Answer from the drawing. Dimensions are ordinates in mm from the lowest x, y and z of the part. A direction names the side the tool comes from. Give positions to 0.01 mm unless a question says otherwise; leave off trailing zeros. Loops run counter-clockwise (first coordinate to the right, second up) from the corner with the lowest first, then second, coordinate; pieces in that order, holes last.
Item 1: A tool of negligible diameter and unlimited length cuts with its end or side. For the marked faces 4 and 5, from which of +Z, -Z, +X, -X, +Y, -Y can it reach the whole face along a straight path? Write none if from no direction.
Item 2: Section B-B, the plane y = 58.5 is taken. Give the vertices of the cut face in (x, z).
Item 3: Consider line 1 along Y through (x, z) = (2.25, 8); line 2 along Z through (x, y) = (4.75, 51.5); line 3 along Z through (x, y) = (9.5, 40.5). Determine where each line is inside the solid, lowest interval first.
Item 4: Each of these flat-tipped pins is pushed along its axis until it touches: pin 1 Ø4 at (y, z) = (68.5, 6.5) entering from +X; pin 2 Ø3 at (y, z) = (51.5, 2) entering from +X; pin 3 Ø1 at (y, z) = (59.5, 1.5) entering from +X. Where does it stop, or does it pass through?
Item 5: Section A-A, the plane z = 5 is taken. Give the vertices of the cut face in (x, y), and give its area (3 significant figures).
Item 6: The mould has two halves that part along Y. Classify the marked faces 1, 2 and 3: pulls with the +Y half, pulls with the -Y half, needs draft (parallel to the pull), parting line crosses it, or undercut.
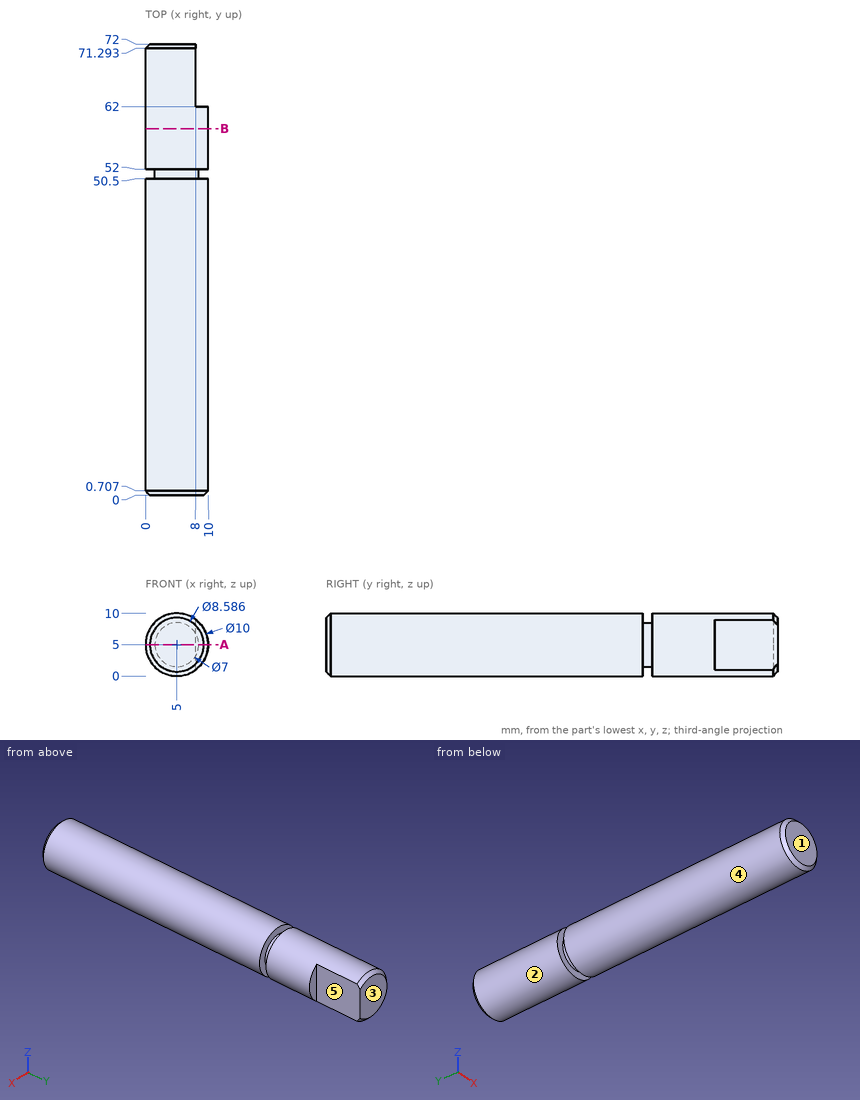
Worked answers:
1. face 4: +Y, -Y
1. face 5: +Z, -Z, +X, +Y
2. outline: circle Ø10 at (5, 5)
3. line 1: y = 0 to 50.5, 52 to 72
3. line 2: z = 1.51 to 8.49
3. line 3: z = 2.82 to 7.18
4. pin 1: stops at x = 8
4. pin 2: stops at x = 9.74
4. pin 3: stops at x = 9
5. outline: (0, 0.71) - (0.71, 0) - (9.29, 0) - (10, 0.71) - (10, 50.5) - (8.5, 50.5) - (8.5, 52) - (10, 52) - (10, 62) - (8, 62) - (8, 72) - (0.71, 72) - (0, 71.29) - (0, 52) - (1.5, 52) - (1.5, 50.5) - (0, 50.5) - close
5. area: 695 mm2
6. face 1: pulls with the -Y half
6. face 2: needs draft
6. face 3: pulls with the +Y half
